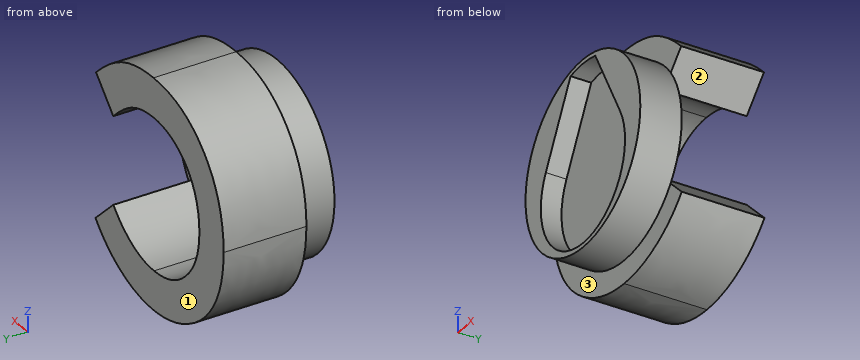
```python
from build123d import *

# Parameters (mm, degrees)
SKETCH1_R           = 22.5
BOSS_EXTRUDE1_DEPTH = 10
BOSS_EXTRUDE2_DEPTH = 20
SKETCH3_R           = 16.5
CUT_EXTRUDE2_DEPTH  = 5


with BuildPart() as part:
    # Sketch1 → Boss-Extrude1 (new body)
    with BuildSketch(Plane(origin=(0, 0, 0), x_dir=(1, 0, 0), z_dir=(0, 1, 0))):
        with Locations(Location((0, 0, 0), (0, 0, 270))):
            Circle(SKETCH1_R)
    extrude(amount=BOSS_EXTRUDE1_DEPTH)

    # Sketch2 → Boss-Extrude2 (add)
    with BuildSketch(Plane(origin=(0, 10, 0), x_dir=(1, 0, 0), z_dir=(0, 1, 0))):
        with BuildLine():
            Line((22.514356491, 17.490690637), (15.549963462, 10.833706128))
            add(Edge.make_bspline(
                [(15.549963462, 10.833706128), (14.959186907, 11.444570075), (13.805215213, 12.637778742), (11.945732542, 14.217481862), (10.01193827, 15.533950672), (8.041450503, 16.642672321), (5.998825878, 17.481499268), (3.907682699, 18.092766593), (1.754668401, 18.465433177), (0.297591136, 18.508072829), (-0.435279594, 18.529519429)],
                knots=[0, 0, 0, 0, 1.115251505, 2.178435587, 3.19620269, 4.182487026, 5.141301733, 6.088180966, 7.038406374, 8, 8, 8, 8], degree=3))
            add(Edge.make_bspline(
                [(-0.435279594, 18.529519429), (-1.047315714, 18.512575866), (-2.255101565, 18.47913961), (-4.028447695, 18.234018873), (-5.724744916, 17.817180392), (-7.349799924, 17.242699751), (-8.898830923, 16.499352293), (-10.37508565, 15.587713348), (-11.77492446, 14.516016314), (-13.079856293, 13.2898062), (-14.273562073, 11.950079505), (-15.328277138, 10.520594316), (-16.211770191, 9.004625506), (-16.936838569, 7.417525692), (-17.501638807, 5.75194899), (-17.904977137, 4.009016732), (-18.138257248, 2.186653221), (-18.173075868, 0.947824086), (-18.190771715, 0.318214675)],
                knots=[0, 0, 0, 0, 1.035432265, 2.043311493, 3.022114605, 3.98653278, 4.95457646, 5.923598177, 6.917315552, 7.932509744, 8.948865224, 9.949768934, 10.933144597, 11.912367597, 12.897413939, 13.903909035, 14.934704909, 16, 16, 16, 16], degree=3))
            add(Edge.make_bspline(
                [(-18.190771715, 0.318214675), (-18.185671973, -0.123689261), (-18.175620278, -0.994691), (-18.065586703, -2.283144309), (-17.888406699, -3.533248623), (-17.631983338, -4.743110368), (-17.311323403, -5.91377802), (-16.935116286, -7.055350871), (-16.463169991, -8.152054953), (-15.939302484, -9.216627772), (-15.330050609, -10.220021127), (-14.673164696, -11.176839965), (-13.960879171, -12.082394056), (-13.188580519, -12.932981467), (-12.345399597, -13.715309421), (-11.453129512, -14.452903451), (-10.496718903, -15.127299081), (-9.496034842, -15.75542101), (-8.442432682, -16.301075874), (-7.364499094, -16.795333764), (-6.245890431, -17.196744657), (-5.100226426, -17.520318456), (-3.931601279, -17.795469647), (-2.72858475, -17.964888691), (-1.501605485, -18.09318775), (-0.67237345, -18.101109467), (-0.255074599, -18.105095955)],
                knots=[0, 0, 0, 0, 1.103660481, 2.175337485, 3.227646561, 4.255952547, 5.262355991, 6.258840057, 7.255597736, 8.242457506, 9.22035537, 10.185017736, 11.140346927, 12.096287581, 13.051739095, 14.01125915, 14.986044842, 15.97314143, 16.960198552, 17.947847494, 18.933482797, 19.925264591, 20.920966487, 21.929612487, 22.958107872, 24, 24, 24, 24], degree=3))
            add(Edge.make_bspline(
                [(-0.255074599, -18.105095955), (0.452735966, -18.084622318), (1.843399669, -18.044396943), (3.884398613, -17.729840213), (5.829267273, -17.212412193), (7.383208025, -16.601359767), (8.600679559, -15.997937564), (9.52752264, -15.439801741), (10.485950624, -14.815465543), (11.460044841, -14.101365846), (12.460761919, -13.306072133), (13.470436894, -12.412165987), (14.514917625, -11.449082455), (15.199146599, -10.761710818), (15.549963462, -10.409282654)],
                knots=[0, 0, 0, 0, 1.404581149, 2.759636711, 4.088442092, 5.392261763, 6.066678138, 6.783632037, 7.538459478, 8.336747902, 9.180226004, 10.074962426, 11.012997595, 12, 12, 12, 12], degree=3))
            Line((15.549963462, -10.409282654), (22.302350615, -17.500879208))
            add(Edge.make_bspline(
                [(22.302350615, -17.500879208), (21.827694143, -17.95914513), (20.901266219, -18.853582206), (19.503775414, -20.12359939), (18.108043407, -21.264851013), (16.747788174, -22.318759505), (15.400727318, -23.254621954), (14.067003691, -24.073373015), (12.761715627, -24.795720088), (11.457758402, -25.409481144), (10.147018122, -25.930628026), (8.798420406, -26.379301284), (7.407842465, -26.75886272), (5.966791283, -27.06511895), (4.488708107, -27.310695102), (2.959760044, -27.476457584), (1.389641377, -27.587894186), (0.324605561, -27.597907688), (-0.212673424, -27.602959203)],
                knots=[0, 0, 0, 0, 1.244526981, 2.429050516, 3.560637417, 4.644440555, 5.67424972, 6.652764056, 7.595344123, 8.486817594, 9.369275933, 10.254498637, 11.166417451, 12.086725134, 13.032340136, 13.991389299, 14.986715468, 16, 16, 16, 16], degree=3))
            add(Edge.make_bspline(
                [(-0.212673424, -27.602959203), (-1.199588367, -27.577800773), (-3.130706581, -27.528572719), (-5.960709972, -27.163826165), (-8.649137226, -26.552334995), (-11.202528785, -25.687517816), (-13.620072728, -24.582754401), (-15.901150575, -23.22836633), (-18.042085734, -21.627951998), (-20.025583664, -19.800269815), (-21.819751941, -17.781748276), (-23.405588922, -15.614409906), (-24.717393333, -13.287603029), (-25.806612801, -10.835702017), (-26.658368101, -8.247517893), (-27.257859435, -5.520251029), (-27.627561366, -2.656534771), (-27.668007283, -0.700550553), (-27.688634962, 0.297014088)],
                knots=[0, 0, 0, 0, 1.078019885, 2.10938526, 3.111377082, 4.085535484, 5.04941344, 6.010039228, 6.978205633, 7.964457913, 8.951525778, 9.924444315, 10.892603023, 11.863865945, 12.85144698, 13.863884204, 14.910567087, 16, 16, 16, 16], degree=3))
            add(Edge.make_bspline(
                [(-27.688634962, 0.297014088), (-27.679918705, 0.947617235), (-27.662645212, 2.23695366), (-27.481099205, 4.136250673), (-27.228013516, 5.987725528), (-26.826516082, 7.772153781), (-26.342550525, 9.513574972), (-25.74067577, 11.193061886), (-25.021853092, 12.815441538), (-24.20925184, 14.383429889), (-23.289964174, 15.886754934), (-22.263018932, 17.312500744), (-21.154853689, 18.671673812), (-19.93884104, 19.946242185), (-18.632651242, 21.14739682), (-17.230386997, 22.268628432), (-15.740482224, 23.326016746), (-14.158904306, 24.292294284), (-12.516379087, 25.166343676), (-10.833623133, 25.937292571), (-9.114770779, 26.581628309), (-7.367089489, 27.116081037), (-5.583195332, 27.515012207), (-3.775821291, 27.816990234), (-1.929588783, 27.985797881), (-0.690003597, 28.013432771), (-0.064269311, 28.027382677)],
                knots=[0, 0, 0, 0, 1.071919942, 2.124283339, 3.142214191, 4.149696895, 5.136002878, 6.119640489, 7.086990633, 8.058538607, 9.028339693, 9.988281803, 10.952401235, 11.916291999, 12.888973767, 13.874849856, 14.873389453, 15.898127285, 16.927174885, 17.938320013, 18.946391617, 19.950418109, 20.947802303, 21.956882652, 22.968648068, 24, 24, 24, 24], degree=3))
            add(Edge.make_bspline(
                [(-0.064269311, 28.027382677), (0.469546195, 28.019386243), (1.53162701, 28.003476514), (3.113243568, 27.870851616), (4.682211098, 27.662565556), (6.232912213, 27.348306247), (7.776439114, 26.975240735), (9.292508128, 26.486762906), (10.805036063, 25.942262312), (12.290301164, 25.291423032), (13.750376645, 24.580973168), (15.151057936, 23.774941998), (16.515862348, 22.922931778), (17.814546634, 21.974516811), (19.071437948, 20.964097872), (20.279963894, 19.886960788), (21.429518951, 18.725146522), (22.150915876, 17.904256161), (22.514356491, 17.490690637)],
                knots=[0, 0, 0, 0, 0.996412454, 1.982464992, 2.961075852, 3.949442424, 4.934965278, 5.923860011, 6.921385422, 7.934793307, 8.949617135, 9.951082467, 10.950285876, 11.951772932, 12.951063433, 13.960125323, 14.972308753, 16, 16, 16, 16], degree=3))
        make_face()
    extrude(amount=BOSS_EXTRUDE2_DEPTH)

    # Sketch3 → Cut-Extrude2 (cut)
    with BuildSketch(Plane.XZ):
        with BuildLine():
            ThreePointArc((-14.551420086, 2.778571429), (0, 11.5), (14.551420086, 2.778571429))
            Line((14.551420086, 2.778571429), (4.83856504, 20.948467447))
            ThreePointArc((4.83856504, 20.948467447), (0, 21.5), (-4.83856504, 20.948467447))
            Line((-4.83856504, 20.948467447), (-14.551420086, 2.778571429))
        make_face()
        with Locations((0, -5)):
            Circle(SKETCH3_R)
    extrude(amount=-CUT_EXTRUDE2_DEPTH, mode=Mode.SUBTRACT)


solid = part.part
```
The listing builds one solid part. Answer for the finished solid, in the listing's coordinates (mm). Face numbers are marked on the shaded views. A direction names the side the tool comes from. Round coordinates to 2 decimals unless told otherwise and drop trailing zeros. Loops run counter-clockwise (first coordinate to the right, second up) from the corner with the lowest first, then second, coordinate; pieces in that order, holes last.
Q1. Which of the six approach directions +Z, -Z, +X, -X, +Y, -Y give full straight-line access (tool end or side, diameter ignored) to the marked faces 1, 2 and 3?
Q2. Find the intervals of material crossed by line 1 (Y direction, x = 0.5, z = 20.5); line 2 (X direction, y = 2, z = -5); line 3 (Y direction, x = -5.5, z = -15.5), in increasing order.
Q3. Section A-A, the plane y = 3.5 is taken. Determine the outline of the cut face in (x, z).
Q4. Given pin 1 Ø1 at (x, z) = (16.5, 10.5) entering from +Y; pin 2 Ø6 at (x, y) = (-20, 20) entering from -Z; pin 3 Ø8 at (x, y) = (-13.5, 3.5) entering from -Z, each flat-ended and moving along its own axis, determine where each tip first touches the part or whether it passes through.
Completed:
1. face 1: +Z, -Z, +X, -X, +Y
1. face 2: +X, +Y
1. face 3: -Y
2. line 1: y = 5 to 30
2. line 2: x = -21.94 to -16.5, 16.5 to 21.94
2. line 3: y = 5 to 10
3. outline: circle Ø45 at (0, 0); hole (-14.55, 2.78) arc R16.5 ccw (long way) to (14.55, 2.78) - (4.84, 20.95) arc R21.5 ccw to (-4.84, 20.95) - close
4. pin 1: stops at y = 10
4. pin 2: stops at z = -22.42
4. pin 3: stops at z = -20.4
